The model under review builds one solid part; all positions refer to its coordinate system, in mm. A direction names the side the tool comes from. Coordinates: 2 decimals unless noted, no trailing zeros. Loops run counter-clockwise (first coordinate to the right, second up) from the corner with the lowest first, then second, coordinate; pieces in that order, holes last. Notation, with made-up numbers: M 3,66 L 29,66 A16 cw 29,88 Z; hole C -39.5,-18.5 d4. An arc over 180 degrees is marked long. Use CSV: the item, a comma, the result in double quotes. Start each with the question number.
from build123d import *

# Parameters (mm, degrees)
F0_R     = 50
F1_DEPTH = 2
F2_R     = 50
F2_R_2   = 48
F2_R_3   = 43
F2_R_4   = 41
F3_DEPTH = 3
F4_R     = 0.95
F5_DEPTH = 2.001
F6_R     = 10
F7_DEPTH = 2.001


with BuildPart() as f1:
    # F0 (on Top) → F1 (new body)
    with BuildSketch(Plane.XY):
        Circle(F0_R)
    extrude(amount=F1_DEPTH)

    # F2 (on face) → F3 (join)
    with BuildSketch(Plane.XY.offset(2)):
        Circle(F2_R)
        Circle(F2_R_2, mode=Mode.SUBTRACT)
        Circle(F2_R_3)
        Circle(F2_R_4, mode=Mode.SUBTRACT)
    extrude(amount=F3_DEPTH)

    # F4 (on face) → F5 (cut, through all)
    with BuildSketch(Plane.XY.offset(2)):
        with Locations((0, 45.5)):
            Circle(F4_R)
        with Locations((-26.7442289793, 36.8102732441)):
            Circle(F4_R)
        with Locations((-43.2730714914, 14.0602732441)):
            Circle(F4_R)
        with Locations((-43.2730714914, -14.0602732441)):
            Circle(F4_R)
        with Locations((-26.7442289793, -36.8102732441)):
            Circle(F4_R)
        with Locations((0, -45.5)):
            Circle(F4_R)
        with Locations((26.7442289793, -36.8102732441)):
            Circle(F4_R)
        with Locations((43.2730714914, -14.0602732441)):
            Circle(F4_R)
        with Locations((43.2730714914, 14.0602732441)):
            Circle(F4_R)
        with Locations((26.7442289793, 36.8102732441)):
            Circle(F4_R)
    extrude(amount=-F5_DEPTH, mode=Mode.SUBTRACT)

    # F6 (on face) → F7 (cut, through all)
    with BuildSketch(Plane.XY.offset(2)):
        Circle(F6_R)
    extrude(amount=-F7_DEPTH, mode=Mode.SUBTRACT)


solid = f1.part
1. To check wall thickness, follow line 1 along Y through (x, z) = (0, 1.45); line 2 along Y through (x, z) = (7.5, 4.1); line 3 along X through (y, z) = (5.5, 2.5). State the ranges of each line that lie inside material, in increasing order.
2. Add section D-D (y = 29). Write out the cut boundary in (x, z).
3. Add section B-B (z = 4.05). Write out the cut boundary in (x, y), plus the area to 3 significant figures.
4. Insertion check: pin 1 Ø2 at (x, y) = (-26.74, -36.81) entering from +Z; pin 2 Ø3 at (x, z) = (34.5, 3.5) entering from -Y. Each pin has a flat end and moves straight along its axis. Give the tip position at first contact, or say it passes through.
5. Add section A-A (y = 0). Write out the cut boundary in (x, z).
6. Draft analysis for pull direction Y (two halves, no side actions). For faces 1 (the flat face through (-0.7, -10.4, 0)), 2 (the flat face through (-29, 32, 2)), 3 (the cylindrical face through (47.69, 15.02, 2.46)), state which applies: released by +Y, released by -Y, zero draft, split by the parting line, or undercut.
7. For faces 4 (the cylindrical face through (-5.598, 42.634, 3.479)), 5 (the flat face through (38, -16, 5)), list the 3-axis set-ups (+Z, -Z, +X, -X, +Y, -Y) from which the entire face can be reached by the end or side of a thin tool; tool diameter is ignored.
8. Add section C-C (x = 32). Write out the cut boundary in (y, z).
Solved:
1,line 1,"y = -50 to -46.45, -44.55 to -10, 10 to 44.55, 46.45 to 50"
1,line 2,"y = -49.43 to -47.41, -42.34 to -40.31, 40.31 to 42.34, 47.41 to 49.43"
1,line 3,"x = -49.7 to -47.68, -42.65 to -40.63, 40.63 to 42.65, 47.68 to 49.7"
2,outline,"M -40.73,0 L 40.73,0 L 40.73,5 L 38.25,5 L 38.25,2 L 31.75,2 L 31.75,5 L 28.98,5 L 28.98,2 L -28.98,2 L -28.98,5 L -31.75,5 L -31.75,2 L -38.25,2 L -38.25,5 L -40.73,5 Z"
3,outline,"C 0,0 d100; C 0,0 d86; hole C 0,0 d96; hole C 0,0 d82"
3,area,"1,140 mm^2"
4,pin 1,"stops at z = 2"
4,pin 2,"stops at y = -37.56"
5,outline,"M -50,0 L -10,0 L -10,2 L -41,2 L -41,5 L -43,5 L -43,2 L -48,2 L -48,5 L -50,5 Z; M 10,0 L 50,0 L 50,5 L 48,5 L 48,2 L 43,2 L 43,5 L 41,5 L 41,2 L 10,2 Z"
6,face 1,"zero draft"
6,face 2,"undercut"
6,face 3,"split by the parting line"
7,face 4,"+Z"
7,face 5,"+Z, +X, -X, +Y, -Y"
8,outline,"M -38.42,0 L 38.42,0 L 38.42,5 L 35.78,5 L 35.78,2 L 28.72,2 L 28.72,5 L 25.63,5 L 25.63,2 L -25.63,2 L -25.63,5 L -28.72,5 L -28.72,2 L -35.78,2 L -35.78,5 L -38.42,5 Z"
